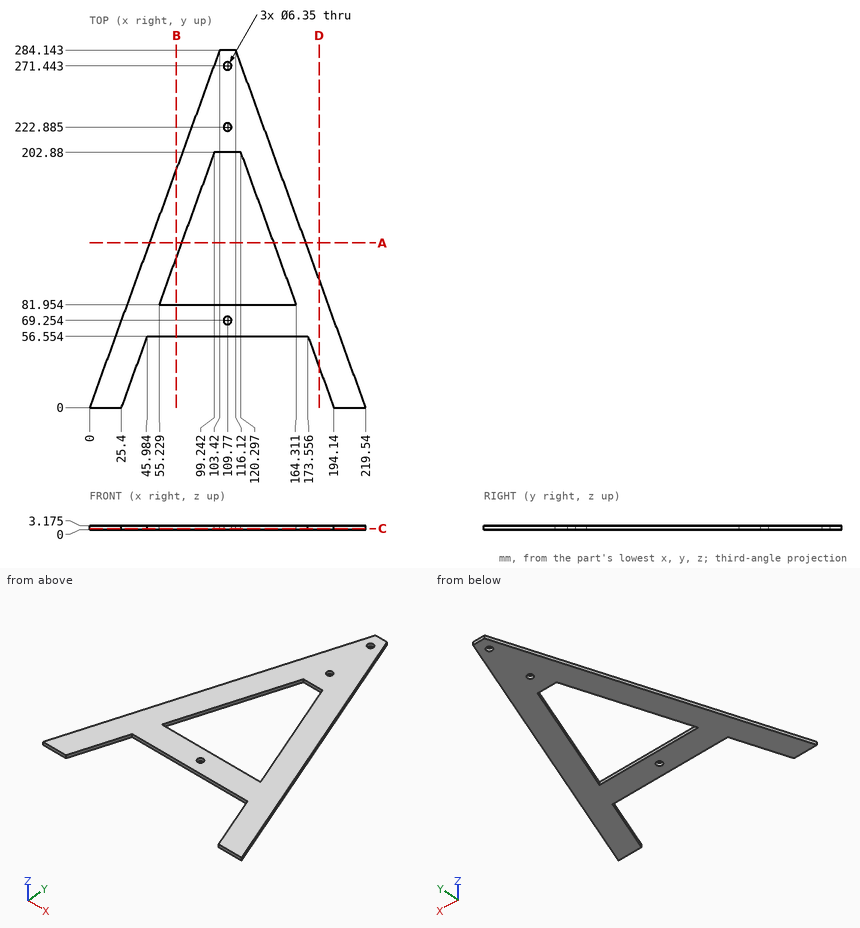
Drawing for the job (mm, zero at the part's lowest x, y, z). Round coordinates to 2 decimals unless told otherwise and drop trailing zeros. Order: outer loops, then holes, each group sorted by start corner. A loop starts at its lowest first (then second) coordinate and runs counter-clockwise, first axis right, second up. Notation, with made-up numbers: M -31.5,82 L -9.5,82 A15 ccw -9.5,107 Z; hole C 24,16 d6. An arc over 180 degrees is marked long. Use one line per item in the form item = value.
Q1. Saw through at A-A on y = 131. Give the cut face in (x, z) (1 decimal), then the cut area to 3 significant figures.
Recorded:
outline = M 47.7,0 L 73.1,0 L 73.1,3.2 L 47.7,3.2 Z; M 146.5,0 L 171.9,0 L 171.9,3.2 L 146.5,3.2 Z
area = 161 mm^2
Q2. Saw through at B-B on x = 69. Give the cut face in (y, z) (1 decimal), then the cut area to 3 significant figures.
Recorded:
outline = M 56.6,0 L 82,0 L 82,3.2 L 56.6,3.2 Z; M 119.8,0 L 189.6,0 L 189.6,3.2 L 119.8,3.2 Z
area = 302 mm^2
Q3. Flat gauge pin, fed straight in: P1, Ø1.5, axis at x = 58, z = 0.5, coming from the -Y side. Where does the tip first touch, or does it go through?
Recorded:
P1 = 56.55
Q4. Saw through at D-D on x = 182.5. Give the cut face in (y, z) (1 decimal).
Recorded:
outline = M 32,0 L 101.8,0 L 101.8,3.2 L 32,3.2 Z
Q5. Saw through at C-C on z = 0.9. State how many separate pieces and enclosed holes the cut face has, then the cut area to 3 significant figures.
Recorded:
separate_pieces = 1
enclosed_holes = 4
area = 16,700 mm^2
Q6. Probe L1, parallel to Y at x = 106, z = 0.8; L2, parallel to X at y = 150.5, z = 1.95; L3, parallel to X at y = 69, z = 2.2 (1 decimal). List the from-to ranges inside material, lowest first.
Recorded:
L1 = 56.55 to 81.95, 202.88 to 284.14
L2 = 54.78 to 80.18, 139.36 to 164.76
L3 = 25.1 to 106.6, 112.9 to 194.4
